For this review, take the finished solid that the model builds, in its own axes (mm). Face numbers are marked on the shaded views. Coordinates: 2 decimals unless noted, no trailing zeros. Loops run counter-clockwise (first coordinate to the right, second up) from the corner with the lowest first, then second, coordinate; pieces in that order, holes last. Notation, with made-up numbers: (27.25, -11) -> (47.25, -11) arc R13 ccw to (47.25, -1) -> close; hole circle Ø7 at (75, 63.25). An arc over 180 degrees is marked (long way). Use a Markdown table: item, result.
Autodesk Inventor part; units mm, degrees
ref_plane "YZ Plane" through (0, 0, 0) normal (1, 0, 0) x (0, 1, 0)
ref_plane "XZ Plane" through (0, 0, 0) normal (0, 1, 0) x (-1, 0, 0)
ref_plane "XY Plane" through (0, 0, 0) normal (0, 0, 1) x (1, 0, 0)
sketch "плоскость" plane through (0, 0, 0) normal (0, 1, 0) x (-1, 0, 0)
  line L0 (0, 0) -> (44, 0)
  line L1 (44, 0) -> (44, -106)
  line L2 (44, -106) -> (0, -106)
  line L3 (0, -106) -> (0, 0)
  dimension "d0" = 106
  dimension "d1" = 44
extrude "Выдавливание1" add sketch "плоскость" along normal blind 1.5
sketch "Эскиз2" plane through (0, 1.5, 0) normal (0, 1, 0) x (1, 0, 0)
  line L0 (-41.9, 2.1) -> (-2.1, 2.1)
  line L1 (-2.1, 2.1) -> (-2.1, 103.9)
  line L2 (-2.1, 103.9) -> (-41.9, 103.9)
  line L3 (-41.9, 103.9) -> (-41.9, 2.1)
  line L4 (-44, 0) -> (0, 0)
  line L5 (-44, 106) -> (-44, 0)
  dimension "d4" = 39.8
  dimension "d5" = 101.8
  dimension "d6" = 2.1
  dimension "d20" = 2.1
extrude "Выдавливание2" add sketch "Эскиз2" along normal blind 4
sketch "Эскиз3" plane through (0, 5.5, 0) normal (0, 1, 0) x (1, 0, 0)
  line L0 (-40.9, 3.1) -> (-2.9, 3.1)
  line L1 (-2.9, 3.1) -> (-2.9, 103.1)
  line L2 (-2.9, 103.1) -> (-40.9, 103.1)
  line L3 (-40.9, 103.1) -> (-40.9, 3.1)
  line L4 (-41.9, 103.9) -> (-41.9, 2.1)
  line L5 (-41.9, 2.1) -> (-2.1, 2.1)
  point P0 (0, 0)
  dimension "d10" = 38
  dimension "d11" = 100
  dimension "d12" = 1
  dimension "d13" = 1
extrude "Выдавливание3" cut sketch "Эскиз3" against normal blind 4
sketch "Эскиз7" plane through (-2.1, 1.5, -2.1) normal (1, 0, 0) x (0, 0, -1)
  line L0 (101, 4) -> (1, 4)
  line L1 (66.3, 3.8) -> (46, 3.8)
  line L2 (46, 3.8) -> (46, 4)
  line L3 (46, 4) -> (66.3, 4)
  line L4 (66.3, 4) -> (66.3, 3.8)
  line L5 (101.8, 0) -> (101.8, 4)
  point P0 (-2.1, -1.5)
  point P1 (66.3, 4)
  point P2 (101.8, 2)
  point P3 (66.3, 3.9)
  point P4 (51, 4)
  dimension "d18" = 35.5
  dimension "d19" = 0.2
extrude "Выдавливание4" cut sketch "Эскиз7" against normal blind 2
properties part number "roller_deck_01_10_2025"
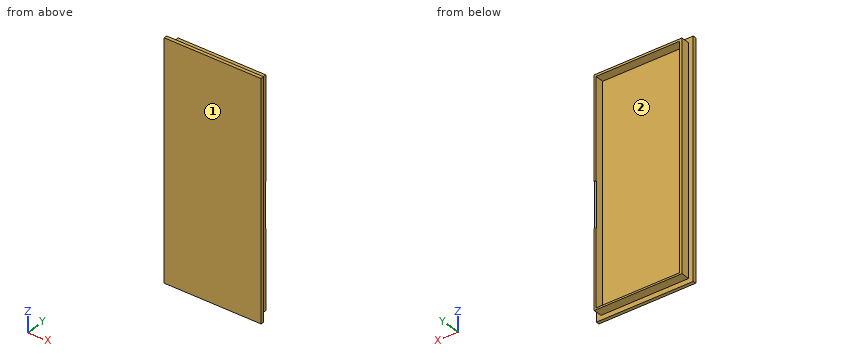
(1) Take a section at B-B on z = -89. Write out the cut boundary in (x, y), plus the area to 3 significant figures.
Found:
| item | result |
|---|---|
| outline | (-44, 0) -> (0, 0) -> (0, 1.5) -> (-2.1, 1.5) -> (-2.1, 5.5) -> (-2.9, 5.5) -> (-2.9, 1.5) -> (-40.9, 1.5) -> (-40.9, 5.5) -> (-41.9, 5.5) -> (-41.9, 1.5) -> (-44, 1.5) -> close |
| area | 73.2 mm^2 |
(2) For pin 1 Ø0.9 at (x, z) = (-2.5, -56) entering from +Y; pin 2 Ø2 at (x, y) = (-31, 3.5) entering from -Z; pin 3 Ø1.5 at (y, z) = (3, -65.5) entering from +X; pin 4 Ø1.5 at (y, z) = (1, -32) entering from +X, all flat-tipped, find the tip position at first contact; note any pin that passes through.
Found:
| item | result |
|---|---|
| pin 1 | stops at y = 5.3 |
| pin 2 | stops at z = -103.9 |
| pin 3 | stops at x = -2.1 |
| pin 4 | stops at x = 0 |
(3) Mouldability with a two-part tool opening along X and no side actions: class the marked faces 1 and 2 as pulls with the +X half, pulls with the -X half, needs draft (parallel to the pull), parting line crosses it, or undercut.
Found:
| item | result |
|---|---|
| face 1 | needs draft |
| face 2 | undercut |
(4) Take a section at C-C on x = -31. Write out the cut boundary in (y, z).
Found:
| item | result |
|---|---|
| outline | (0, -106) -> (1.5, -106) -> (1.5, -103.9) -> (5.5, -103.9) -> (5.5, -103.1) -> (1.5, -103.1) -> (1.5, -3.1) -> (5.5, -3.1) -> (5.5, -2.1) -> (1.5, -2.1) -> (1.5, 0) -> (0, 0) -> close |
(5) For line 1 along Z through (x, y) = (-29.5, 2.4); line 2 along X through (y, z) = (4.1, -58); line 3 along Y through (x, z) = (-38.5, -49), list the stretches that pass through material, from the lowest coordinate up.
Found:
| item | result |
|---|---|
| line 1 | z = -103.9 to -103.1, -3.1 to -2.1 |
| line 2 | x = -41.9 to -40.9, -2.9 to -2.1 |
| line 3 | y = 0 to 1.5 |
(6) Take a section at A-A on y = 4.2. Write out the cut boundary in (x, z), plus the area to 3 significant figures.
Found:
| item | result |
|---|---|
| outline | (-41.9, -103.9) -> (-2.1, -103.9) -> (-2.1, -2.1) -> (-41.9, -2.1) -> close; hole (-40.9, -103.1) -> (-2.9, -103.1) -> (-2.9, -3.1) -> (-40.9, -3.1) -> close |
| area | 252 mm^2 |
